Can you work these out from the model? Positions are in its coordinate system, mm. Face numbers are marked on the shaded views. Round coordinates to 2 decimals unless told otherwise and drop trailing zeros. Write each loop counter-clockwise with the first axis right and the second up, starting at its lowest first coordinate (ties: lowest second). Pieces come first, ordered by that corner, then holes. Notation, with made-up numbers: (71.5, 55.25) -> (98.5, 55.25) arc R14 ccw to (98.5, 62.25) -> close; hole circle Ø9 at (78, 89.5). An arc over 180 degrees is marked (long way). Write item = value, one per line. Start each with the question number.
1) Imagine slicing it at A-A, the plane y = 0. Please give me the cut outline in (x, z).
2) Imagine slicing it at C-C, the plane z = 0. Please give me the cut outline in (x, y).
3) Thinking about a two-plate mould opening in X: for the marked faces 1, 2, 3 and 4, which applies, +X half, -X half, draft (parallel to the pull), parting line (faces both ways), or undercut?
4) Imagine slicing it at B-B, the plane x = 12.7. Please give me the cut outline in (y, z).
5) Imagine slicing it at D-D, the plane y = 6. Please give me the cut outline in (x, z).
6) If I drill on line 1 (Y direction, x = 12.7, z = 6); line 2 (Z direction, x = 20, y = -4.75); line 3 (Y direction, x = 12.7, z = 23.6), over which ranges is the centre line in solid material (lowest first)?
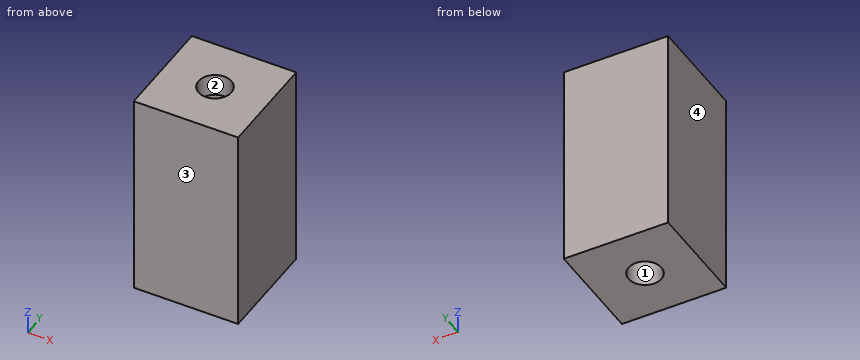
from build123d import *

# Parameters (mm, degrees)
SKETCH1_W           = 50.8
SKETCH1_H           = 25.4
BOSS_EXTRUDE1_DEPTH = 25.4
SKETCH2_R           = 4
CUT_EXTRUDE1_DEPTH  = 50.8
SKETCH3_W           = 10
SKETCH3_H           = 38.541538457


with BuildPart() as part:
    # Sketch1 → Boss-Extrude1 (new body)
    with BuildSketch(Plane(origin=(0, 0, 0), x_dir=(0, 0, -1), z_dir=(1, 0, 0))):
        Rectangle(SKETCH1_W, SKETCH1_H)
    extrude(amount=BOSS_EXTRUDE1_DEPTH)

    # Sketch2 → Cut-Extrude1 (cut)
    with BuildSketch(Plane(origin=(0, 0, -25.4), x_dir=(-1, 0, 0), z_dir=(0, 0, -1))):
        with Locations((-12.7, 0)):
            Circle(SKETCH2_R)
    extrude(amount=-CUT_EXTRUDE1_DEPTH, mode=Mode.SUBTRACT)

    # Sketch3 → Cut-Revolve2 (revolve, cut)
    with BuildSketch(Plane(origin=(0, 0, 0), x_dir=(1, 0, 0), z_dir=(0, 1, 0)), mode=Mode.PRIVATE) as cut_revolve2_sk:
        with Locations((17.7, -0.758930583)):
            Rectangle(SKETCH3_W, SKETCH3_H)
    revolve(cut_revolve2_sk.sketch.rotate(Axis((12.7, 0, 25.4), (0, 0, -1)), 180), axis=Axis((12.7, 0, 25.4), (0, 0, -1)), mode=Mode.SUBTRACT)


solid = part.part
Reported:
q1.outline = (0, -25.4) -> (8.7, -25.4) -> (8.7, -18.51) -> (2.7, -18.51) -> (2.7, 20.03) -> (8.7, 20.03) -> (8.7, 25.4) -> (0, 25.4) -> close; (16.7, -25.4) -> (25.4, -25.4) -> (25.4, 25.4) -> (16.7, 25.4) -> (16.7, 20.03) -> (22.7, 20.03) -> (22.7, -18.51) -> (16.7, -18.51) -> close
q2.outline = (0, -12.7) -> (25.4, -12.7) -> (25.4, 12.7) -> (0, 12.7) -> close; hole circle Ø20 at (12.7, 0)
q3.face_1 = undercut
q3.face_2 = undercut
q3.face_3 = draft
q3.face_4 = -X half
q4.outline = (-12.7, -25.4) -> (-4, -25.4) -> (-4, -18.51) -> (-10, -18.51) -> (-10, 20.03) -> (-4, 20.03) -> (-4, 25.4) -> (-12.7, 25.4) -> close; (4, -25.4) -> (12.7, -25.4) -> (12.7, 25.4) -> (4, 25.4) -> (4, 20.03) -> (10, 20.03) -> (10, -18.51) -> (4, -18.51) -> close
q5.outline = (0, -25.4) -> (25.4, -25.4) -> (25.4, 25.4) -> (0, 25.4) -> close; hole (4.7, -18.51) -> (20.7, -18.51) -> (20.7, 20.03) -> (4.7, 20.03) -> close
q6.line_1 = -12.7 to -10, 10 to 12.7
q6.line_2 = -25.4 to -18.51, 20.03 to 25.4
q6.line_3 = -12.7 to -4, 4 to 12.7
